For this review, take the finished solid that the model builds, in its own axes (mm). A direction names the side the tool comes from. Coordinates: 2 decimals unless noted, no trailing zeros. Loops run counter-clockwise (first coordinate to the right, second up) from the corner with the lowest first, then second, coordinate; pieces in that order, holes last. Notation, with made-up numbers: (-35, 46.5) -> (-6, 46.5) arc R25 ccw to (-6, 67.5) -> close; hole circle Ø4 at (43, 23). An arc over 180 degrees is marked (long way). One line per item, written item: value.
from build123d import *

# Parameters (mm, degrees)
F0_W     = 1828.8
F0_H     = 914.4
F1_DEPTH = 50.8
F2_W     = 50.8
F2_H     = 50.8
F3_DEPTH = 1016


with BuildPart() as f1:
    # F0 (on Top) → F1 (new body)
    with BuildSketch(Plane.XY):
        Rectangle(F0_W, F0_H)
    extrude(amount=F1_DEPTH)

    # F2 (on face) → F3 (join)
    with BuildSketch(Plane.XY.offset(50.8)):
        with Locations((-838.2, -381)):
            Rectangle(F2_W, F2_H)
    extrude(amount=-F3_DEPTH)

    # F4: F1 across plane


with BuildPart() as f1_1:
    add(f1.part)
    add(f1.part.mirror(Plane.XZ))

    # F5: F1 across plane


with BuildPart() as f1_2:
    add(f1_1.part)
    add(f1_1.part.mirror(Plane.YZ))


solid = f1_2.part
1. Insertion check: pin 1 Ø15 at (y, z) = (-378.5, -355) entering from +X; pin 2 Ø1 at (x, y) = (-595, -51) entering from -Z; pin 3 Ø15 at (y, z) = (-375, -610.5) entering from -X. Each pin has a flat end and moves straight along its axis. Give the tip position at first contact, or say it passes through.
Return value:
pin 1: stops at x = 863.6
pin 2: stops at z = 0
pin 3: stops at x = -863.6
2. For faces 1 (the flat face through (-839, 406.4, -476)), 2 (the flat face through (812.8, -381, -476)), 3 (the flat face through (839, -355.6, -476)), 4 (the flat face through (863.6, 381, -476)), list the 3-axis set-ups (+Z, -Z, +X, -X, +Y, -Y) from which the entire face can be reached by the end or side of a thin tool; tool diameter is ignored.
Return value:
face 1: -Z, +X, -X, +Y
face 2: -Z, +Y, -Y
face 3: -Z, +X, -X
face 4: -Z, +X, +Y, -Y
3. Take a section at B-B, the plane x = 794. Give the boundary of the cut face in (y, z).
Return value:
outline: (-457.2, 0) -> (457.2, 0) -> (457.2, 50.8) -> (-457.2, 50.8) -> close
4. Take a section at C-C, the plane y = 190. Give the boundary of the cut face in (x, z), and give its area (3 significant figures).
Return value:
outline: (-914.4, 0) -> (914.4, 0) -> (914.4, 50.8) -> (-914.4, 50.8) -> close
area: 92,900 mm2
5. To check wall thickness, follow probe 1 along Y at (x, z) = (815.5, -346.5); probe 2 along Z at (x, y) = (-629.5, -162.5); probe 3 along X at (y, z) = (-367, -118). State the ranges of each line that lie inside material, in increasing order. Write a range as from..to.
Return value:
probe 1: y = -406.4..-355.6, 355.6..406.4
probe 2: z = 0..50.8
probe 3: x = -863.6..-812.8, 812.8..863.6
6. Take a section at A-A, the plane z = -824.5. Give the boundary of the cut face in (x, y), and give its area (3 significant figures).
Return value:
outline: (-863.6, -406.4) -> (-812.8, -406.4) -> (-812.8, -355.6) -> (-863.6, -355.6) -> close; (-863.6, 355.6) -> (-812.8, 355.6) -> (-812.8, 406.4) -> (-863.6, 406.4) -> close; (812.8, -406.4) -> (863.6, -406.4) -> (863.6, -355.6) -> (812.8, -355.6) -> close; (812.8, 355.6) -> (863.6, 355.6) -> (863.6, 406.4) -> (812.8, 406.4) -> close
area: 10,300 mm2
7. The part is to be moulded in two halves that separate along Y. For faces 5 (the flat face through (839, 355.6, -476)), 6 (the flat face through (-13, -457.2, 25)), 7 (the flat face through (914.4, -6, 25)), say which applies: pulls with the +Y half, pulls with the -Y half, needs draft (parallel to the pull), parting line crosses it, or undercut.
Return value:
face 5: undercut
face 6: pulls with the -Y half
face 7: needs draft
